from build123d import *

# Parameters (mm, degrees)
BOSS_EXTRUDE1_DEPTH = 10


with BuildPart() as part:
    # Sketch1 → Boss-Extrude1 (new body)
    with BuildSketch(Plane(origin=(0, 0, 0), x_dir=(1, 0, 0), z_dir=(0, 1, 0))):
        with BuildLine():
            Line((3.992189406, 4), (0, 4))
            Line((0, 4), (0, 0))
            Line((0, 0), (3.5, 0))
            Line((3.5, 0), (7.5, 0))
            ThreePointArc((7.5, 0), (20, 12.5), (32.5, 0))
            Line((32.5, 0), (36.5, 0))
            Line((36.5, 0), (40, 0))
            Line((40, 0), (40, 4))
            Line((40, 4), (36.007810594, 4))
            ThreePointArc((36.007810594, 4), (20, 16.5), (3.992189406, 4))
        make_face()
    extrude(amount=BOSS_EXTRUDE1_DEPTH)


solid = part.part
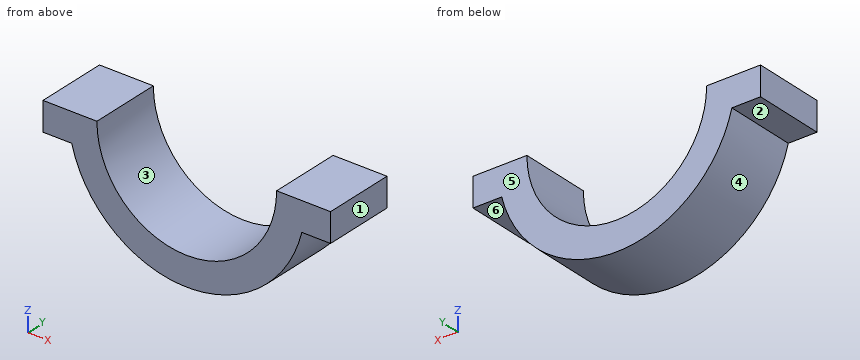
Verification items for the finished model (mm, model axes). Face numbers are marked on the shaded views. A direction names the side the tool comes from. Give positions to 0.01 mm unless a question says otherwise; leave off trailing zeros. Order: outer loops, then holes, each group sorted by start corner. A loop starts at its lowest first (then second) coordinate and runs counter-clockwise, first axis right, second up. Notation, with made-up numbers: (34.25, -19) -> (92.25, -19) arc R19 ccw to (92.25, 0) -> close; hole circle Ø9 at (-17.5, 23). An arc over 180 degrees is marked (long way). Answer as CSV lines item,"result".
Q1. Sectioned sample at B-B on y = 4. Record the cut outline in (x, z).
Solutions:
outline,"(0, -4) -> (3.99, -4) arc R16.5 ccw to (36.01, -4) -> (40, -4) -> (40, 0) -> (32.5, 0) arc R12.5 cw to (7.5, 0) -> (0, 0) -> close"
Q2. Access from +Z, -Z, +X, -X, +Y, -Y to the whole of each face (thin tool, end or side, straight path). Record for the marked faces 5 and 6.
Solutions:
face 5,"+Z, -Z, +X, -X, +Y"
face 6,"-Z, +X, +Y, -Y"
Q3. Sectioned sample at A-A on z = -3. Record the cut outline in (x, y), plus the area to 3 significant figures.
Solutions:
outline,"(0, 0) -> (7.87, 0) -> (7.87, 10) -> (0, 10) -> close; (32.13, 0) -> (40, 0) -> (40, 10) -> (32.13, 10) -> close"
area,"157 mm²"
Q4. Depth check by flat-ended pin: pin 1 (4 mm diameter, centred on y = 5, z = -6.5, fed in from -X); pin 2 (4.5 mm diameter, centred on x = 38.5, y = 7, fed in from -Z); pin 3 (1.5 mm diameter, centred on y = 6, z = -8, fed in from +X). Enter the tip coordinate at first touch or a pass-through.
Solutions:
pin 1,"stops at x = 4.13"
pin 2,"stops at z = -4"
pin 3,"stops at x = 34.82"
Q5. Sectioned sample at C-C on z = -10. Record the cut outline in (x, y).
Solutions:
outline,"(6.88, 0) -> (12.5, 0) -> (12.5, 10) -> (6.88, 10) -> close; (27.5, 0) -> (33.12, 0) -> (33.12, 10) -> (27.5, 10) -> close"
Q6. Sectioned sample at D-D on x = 20. Record the cut outline in (y, z), plus the area to 3 significant figures.
Solutions:
outline,"(0, -16.5) -> (10, -16.5) -> (10, -12.5) -> (0, -12.5) -> close"
area,"40.0 mm²"
Q7. Scan lines: probe 1 along X at (y, z) = (2.5, -2); probe 2 along X at (y, z) = (9, -5.25); probe 3 along Z at (x, y) = (19, 3). Record each from-to range of solid material in increasing order.
Solutions:
probe 1,"x = 0 to 7.66, 32.34 to 40"
probe 2,"x = 4.36 to 8.66, 31.34 to 35.64"
probe 3,"z = -16.47 to -12.46"
Q8. Release check for a two-part mould opening along X. For the marked faces 1, 2, 3 and 4 record: +X half, -X half, draft (parallel to the pull), parting line (faces both ways), or undercut.
Solutions:
face 1,"+X half"
face 2,"draft"
face 3,"undercut"
face 4,"parting line"
